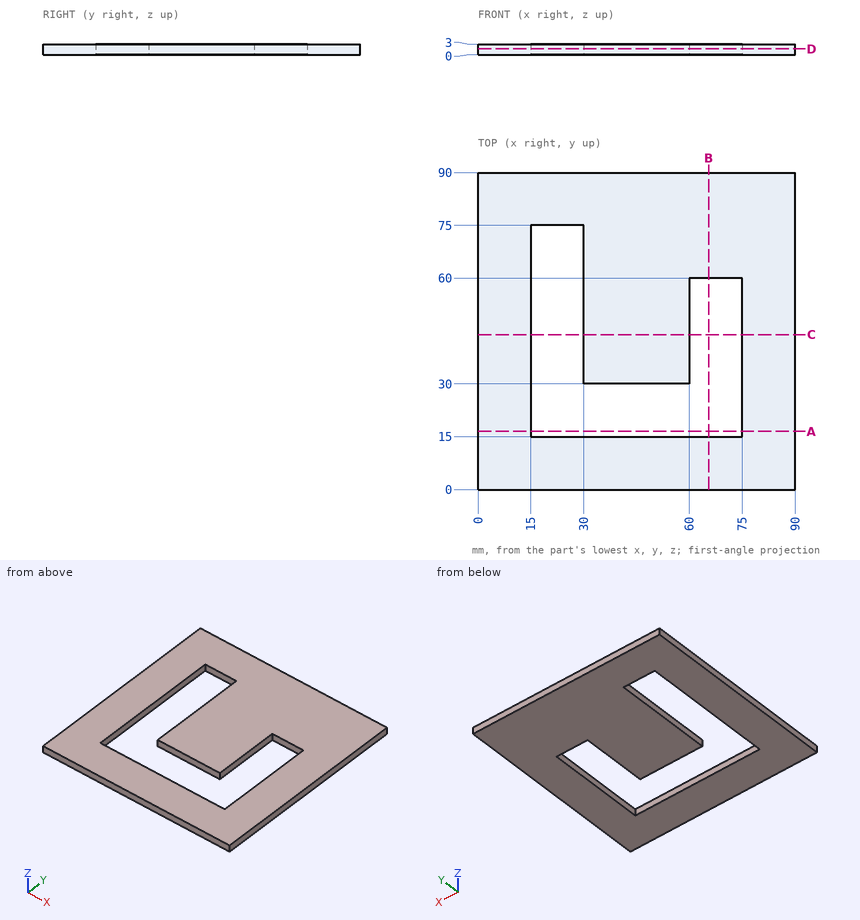
Verification items for this drawing (mm, ordinates from the low corner). Coordinates: 2 decimals unless noted, no trailing zeros. Write each loop counter-clockwise with the first axis right and the second up, starting at its lowest first coordinate (ties: lowest second). Pieces come first, ordered by that corner, then holes. Notation, with made-up numbers: M 65.25,77 L 74.25,77 A10 ccw 74.25,90 Z; hole C 79.25,16.5 d8. An arc over 180 degrees is marked long. Use CSV: the item, a comma, the result in double quotes.
Q1. Section check C-C, the plane y = 44. Enter the section's corners in (x, z).
Computed values:
outline,"M 0,0 L 15,0 L 15,3 L 0,3 Z; M 30,0 L 60,0 L 60,3 L 30,3 Z; M 75,0 L 90,0 L 90,3 L 75,3 Z"
Q2. Section check B-B, the plane x = 65.5. Enter the section's corners in (y, z), and give its area (3 significant figures).
Computed values:
outline,"M 0,0 L 15,0 L 15,3 L 0,3 Z; M 60,0 L 90,0 L 90,3 L 60,3 Z"
area,"135 mm²"
Q3. Section check A-A, the plane y = 16.5. Enter the section's corners in (x, z), and give its area (3 significant figures).
Computed values:
outline,"M 0,0 L 15,0 L 15,3 L 0,3 Z; M 75,0 L 90,0 L 90,3 L 75,3 Z"
area,"90.0 mm²"
Q4. Thickness scan on line 1 along X through (y, z) = (53, 1.4); line 2 along Y through (x, z) = (29, 2.45); line 3 along Y through (x, z) = (74.5, 1.3). Record the ranges inside material, lowest first. Write a range as [from, to].
Computed values:
line 1,"[0, 15], [30, 60], [75, 90]"
line 2,"[0, 15], [75, 90]"
line 3,"[0, 15], [60, 90]"
Q5. Section check D-D, the plane z = 1.6. Enter the section's corners in (x, y).
Computed values:
outline,"M 0,0 L 90,0 L 90,90 L 0,90 Z; hole M 15,15 L 75,15 L 75,60 L 60,60 L 60,30 L 30,30 L 30,75 L 15,75 Z"
